The model under review builds one solid part; all positions refer to its coordinate system, in mm. Give positions to 0.01 mm unless a question says otherwise; leave off trailing zeros. Order: outer loops, then holes, each group sorted by start corner. A loop starts at its lowest first (then second) coordinate and runs counter-clockwise, first axis right, second up.
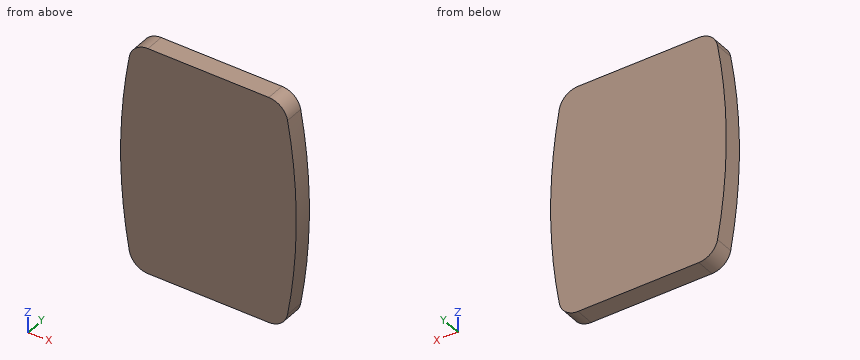
```python
from build123d import *

# Parameters (mm, degrees)
F1_DEPTH = 19.05
F2_DEPTH = 19.05
F3_DEPTH = 19.05
F4_R     = 19.05


with BuildPart() as f1:
    # F0 (on Front) → F1 (new body)
    with BuildSketch(Plane.XZ):
        Polygon((-92.987883, 161.679518), (-113.869874, 161.679518), (-113.869874, -66.920482), (-99.337883, -66.920482), (-92.987883, -66.920482), (-81.616402, -66.920482), (-75.266402, -66.920482), (38.530126, -66.920482), (38.530126, 161.679518), (-81.616402, 161.679518), align=None)
    extrude(amount=F1_DEPTH)

    # F0 (on Front) → F2 (join)
    with BuildSketch(Plane.XZ):
        with BuildLine():
            Line((-113.869874, -66.920482), (-113.869874, 161.679518))
            ThreePointArc((-113.869874, 161.679518), (-125.585738, 47.379518), (-113.869874, -66.920482))
        make_face()
    extrude(amount=F2_DEPTH)

    # F0 (on Front) → F3 (join)
    with BuildSketch(Plane.XZ):
        with BuildLine():
            ThreePointArc((38.530126, -66.920482), (50.245991, 47.379518), (38.530126, 161.679518))
            Line((38.530126, 161.679518), (38.530126, -66.920482))
        make_face()
    extrude(amount=F3_DEPTH)

    # F4
    f4_edges = [f1.edges().sort_by_distance(p)[0] for p in [
        (-113.869874, -9.525, 161.679518),
        (38.530126, -9.525, 161.679518),
        (38.530126, -9.525, -66.920482),
        (-113.869874, -9.525, -66.920482),
    ]]
    fillet(f4_edges, radius=F4_R)


solid = f1.part
```
1. To check wall thickness, follow line 1 (X direction, y = -10.5, z = 52); line 2 (X direction, y = -7.5, z = 54); line 3 (Z direction, x = -106, y = -1.5). State the ranges of each line that lie inside material, in increasing order.
2. Take a section at B-B (z = 2). Write out the cut boundary in (x, y).
3. Insertion check: pin 1 (8 mm diameter, centred on y = -11, z = -7, fed in from -X); pin 2 (4 mm diameter, centred on y = -8, z = 118.5, fed in from -X); pin 3 (3 mm diameter, centred on y = -16, z = 40.5, fed in from +X). Each pin has a flat end and moves straight along its axis. Give the tip position at first contact, or say it passes through.
4. Take a section at C-C (x = 31.5). Write out the cut boundary in (y, z).
5. Take a section at A-A (y = -15.25). Write out the cut boundary in (x, z).
Answer:
1. line 1: x = -125.57 to 50.23
1. line 2: x = -125.55 to 50.21
1. line 3: z = -65.22 to 159.98
2. outline: (-123.76, -19.05) - (48.42, -19.05) - (48.42, 0) - (-123.76, 0) - close
3. pin 1: stops at x = -123.33
3. pin 2: stops at x = -121.33
3. pin 3: stops at x = 50.22
4. outline: (-19.05, -64.82) - (0, -64.82) - (0, 159.58) - (-19.05, 159.58) - close
5. outline: (-116.89, -51.2) arc R19.05 ccw to (-98.14, -66.92) - (22.8, -66.92) arc R19.05 ccw to (41.55, -51.2) arc R563.41 ccw to (41.55, 145.96) arc R19.05 ccw to (22.8, 161.68) - (-98.14, 161.68) arc R19.05 ccw to (-116.89, 145.96) arc R563.41 ccw to start
